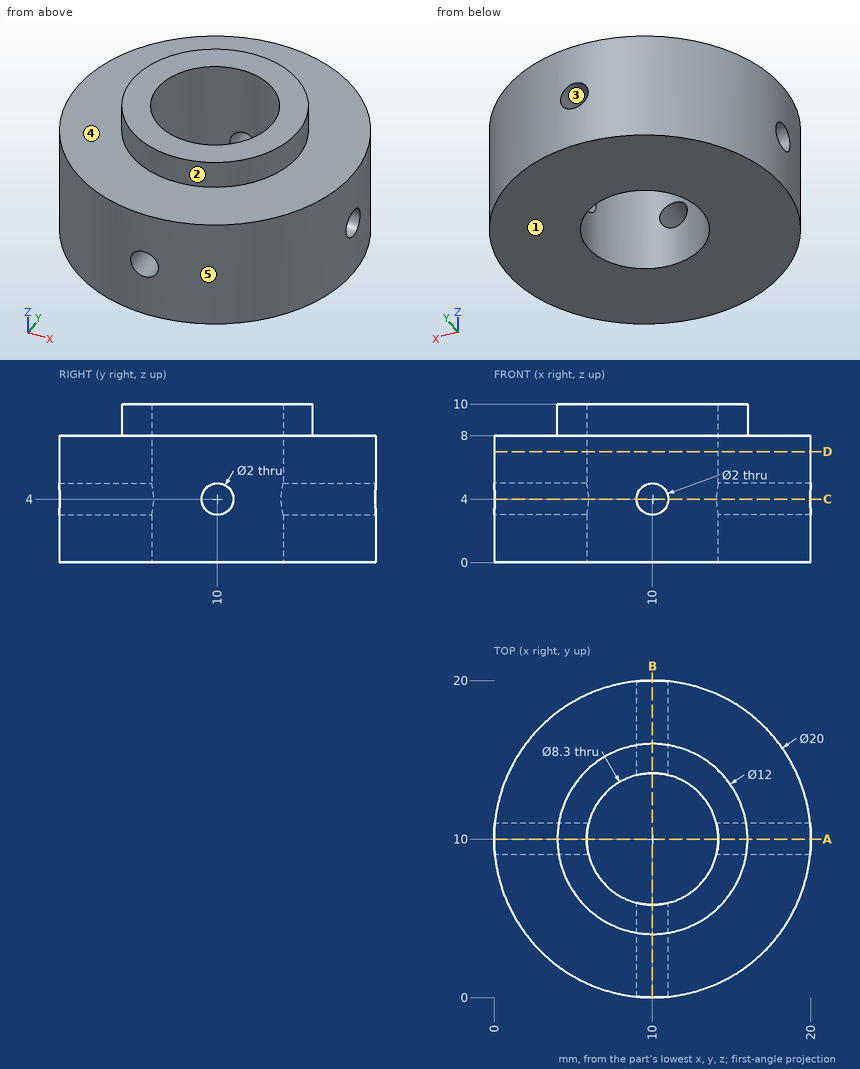
Part print with two shaded views. Sizes in mm from the minimum x, y, z corner. A direction names the side the tool comes from. Give positions to 0.01 mm unless a question says otherwise; leave off trailing zeros. Write each loop counter-clockwise with the first axis right and the second up, starting at its lowest first coordinate (ties: lowest second). Pieces come first, ordered by that corner, then holes.
1) Cut at C-C on z = 4. Write the cut outline in (x, y).
Resolved:
outline: (0.05, 9) arc R10 ccw to (9, 0.05) - (9, 5.97) arc R4.15 cw to (5.97, 9) - close; (0.05, 11) - (5.97, 11) arc R4.15 cw to (9, 14.03) - (9, 19.95) arc R10 ccw to start; (11, 0.05) arc R10 ccw to (19.95, 9) - (14.03, 9) arc R4.15 cw to (11, 5.97) - close; (11, 14.03) arc R4.15 cw to (14.03, 11) - (19.95, 11) arc R10 ccw to (11, 19.95) - close
2) Probe L1, parallel to X at y = 18, z = 4; L2, parallel to Y at x = 10, z = 2.5; L3, parallel to Z at x = 12.5, y = 2.5. List the from-to ranges inside material, lowest first.
Resolved:
L1: x = 4 to 9, 11 to 16
L2: y = 0 to 5.85, 14.15 to 20
L3: z = 0 to 8
3) Cut at D-D on z = 7. Write the cut outline in (x, y).
Resolved:
outline: circle Ø20 at (10, 10); hole circle Ø8.3 at (10, 10)
4) Pin check, flat tips, straight feed: pin 1 (9.5 mm diameter, centred on x = 10, y = 10, fed in from +Z); pin 2 (5 mm diameter, centred on y = 2, z = 5, fed in from +X); pin 3 (1.8 mm diameter, centred on x = 10, z = 4, fed in from -Y); pin 4 (1.5 mm diameter, centred on y = 6.5, z = 2.5, fed in from +X). Stop position of each tip, or through.
Resolved:
pin 1: stops at z = 10
pin 2: stops at x = 18.35
pin 3: passes through
pin 4: stops at x = 19.61
5) Two-plate mould, pull along Z, no slides. Class the marked faces 1, 2 and 3: released by +Z, released by -Z, zero draft, split by the parting line, or undercut.
Resolved:
face 1: released by -Z
face 2: zero draft
face 3: undercut
6) Cut at A-A on y = 10. Write the cut outline in (x, z).
Resolved:
outline: (0, 0) - (5.85, 0) - (5.85, 3) - (0, 3) - close; (0, 5) - (5.85, 5) - (5.85, 10) - (4, 10) - (4, 8) - (0, 8) - close; (14.15, 0) - (20, 0) - (20, 3) - (14.15, 3) - close; (14.15, 5) - (20, 5) - (20, 8) - (16, 8) - (16, 10) - (14.15, 10) - close
7) Which spindle directions (+Z, -Z, +X, -X, +Y, -Y) get a long thin tool onto all of the face, cutting with end or side? Do the marked faces 4 and 5. Say none if no direction does.
Resolved:
face 4: +Z
face 5: +Z, -Z
